Autodesk Inventor part; units mm, degrees
ref_plane "Work Plane1" through (0, 0, -15) normal (0, 0, 1) x (1, 0, 0)
ref_plane "YZ Plane" through (0, 0, 0) normal (1, 0, 0) x (0, 1, 0)
ref_plane "XZ Plane" through (0, 0, 0) normal (0, 1, 0) x (-1, 0, 0)
sketch "Sketch1" plane through (0, 0, 0) normal (0, 0, 1) x (1, 0, 0)
  line L0 (0, 0) -> (25, 0)
  line L1 (25, 0) -> (25, 40)
  line L2 (25, 40) -> (0, 40)
  line L3 (0, 40) -> (0, 0)
  dimension "d1" = 25
  dimension "d2" = 40
  dimension "d3" = 25
extrude "Extrusion1" add sketch "Sketch1" against normal blind 30
sketch "Sketch2" plane through (25, 0, 0) normal (1, 0, 0) x (0, 0, -1)
  line L0 (0, 0) -> (30, 0)
  circle A0 centre (15, 6.56) radius 2.46
extrude "Extrusion2" cut sketch "Sketch2" against normal blind 30
sketch "Sketch3" plane through (0, 0, 0) normal (-1, 0, 0) x (0, 0, 1)
  line L0 (0, 0) -> (-30, 0)
  line L1 (-25.05, 0) -> (-4.95, 0)
  line L2 (-4.95, 0) -> (-4.95, 33.12)
  line L3 (-4.95, 33.12) -> (-25.05, 33.12)
  line L4 (-25.05, 33.12) -> (-25.05, 0)
  dimension "d11" = 20.1
extrude "Extrusion3" cut sketch "Sketch3" against normal blind 20
sketch "Sketch4" plane through (0, 0, 0) normal (0, -1, 0) x (1, 0, 0)
  line L0 (20, -4.95) -> (20, -25.05)
  line L1 (20, -15) -> (25, -15)
  line L2 (25, 0) -> (25, -30)
  line L3 (20, -8.025) -> (25, -8.025)
  line L4 (25, -8.025) -> (25, -21.975)
  line L5 (25, -21.975) -> (20, -21.975)
  line L6 (20, -21.975) -> (20, -8.025)
  line L7 (20, -8.025) -> (25, -21.975) construction
  line L8 (25, -8.025) -> (20, -21.975) construction
  line L9 (25, -12.54) -> (25, -17.46)
  point P0 (0, 0)
  point P1 (22.5, -15)
  dimension "d14" = 13.95
extrude "Extrusion4" add sketch "Sketch4" along normal blind 15
sketch "Sketch5" plane through (20, 0, 0) normal (-1, 0, 0) x (0, 0, 1)
  circle A0 centre (-15, 6.56) radius 2.46
  circle A1 centre (-15, 6.56) radius 4.7025
  circle A2 centre (-15, 6.56) radius 2.46
  circle A3 centre (-15, 6.56) radius 2.46
  point P0 (0, 0)
  dimension "d17" = 9.405
extrude "Extrusion5" cut sketch "Sketch5" against normal blind 2.1
sketch "Sketch6" plane through (25, 0, 0) normal (1, 0, 0) x (0, 0, -1)
  circle A0 centre (15, 6.56) radius 4.7025
  line L0 (15, 6.56) -> (15, 23.56)
  circle A1 centre (15, 23.56) radius 2.46
  point P0 (0, 0)
  dimension "d20" = 17
  dimension "d21" = 4.92
extrude "Extrusion6" cut sketch "Sketch6" against normal blind 10 contours A1
sketch "Sketch7" plane through (20, 0, 0) normal (-1, 0, 0) x (0, 0, 1)
  circle A0 centre (-15, 23.56) radius 2.46
  circle A1 centre (-15, 23.56) radius 4.7025
  point P0 (0, 0)
  dimension "d24" = 9.405
extrude "Extrusion7" cut sketch "Sketch7" against normal blind 2.1
sketch "Sketch9" plane through (25, 0, 0) normal (1, 0, 0) x (0, 0, -1)
  circle A0 centre (15, 6.56) radius 2.46
  circle A1 centre (15, 6.56) radius 2.46
  circle A2 centre (15, 23.56) radius 2.46
  circle A3 centre (15, 23.56) radius 2.46
  line L0 (30, 40) -> (30, 0)
  line L1 (30, 0) -> (30, 40)
  line L2 (30, 40) -> (0, 40)
  line L3 (0, 40) -> (0, 0)
  line L4 (0, 0) -> (8.025, 0)
  line L5 (21.975, 0) -> (21.975, -15)
  line L6 (21.975, -15) -> (8.025, -15)
  line L7 (8.025, -15) -> (8.025, 0)
  line L8 (0, 0) -> (8.025, 0)
  line L9 (21.975, 0) -> (30, 0)
extrude "Extrusion8" add sketch "Sketch9" along normal blind 5
sketch "Sketch10" plane through (0, 40, 0) normal (0, 1, 0) x (1, 0, 0)
  line L0 (0, 30) -> (30, 30)
  line L1 (30, 0) -> (0, 0)
  line L2 (0, 30) -> (30, 30)
  line L3 (30, 30) -> (30, 0)
  line L4 (30, 0) -> (0, 0)
  line L5 (0, 0) -> (0, 30)
extrude "Extrusion9" add sketch "Sketch10" along normal blind 30
sketch "Sketch12" plane through (30, 0, 0) normal (1, 0, 0) x (0, 0, -1)
  circle A0 centre (15, 6.56) radius 2.46
  line L0 (15, 6.56) -> (15, 15.06)
  circle A1 centre (15, 15.06) radius 2.525
  point P0 (0, 0)
  dimension "d31" = 8.5
  dimension "d33" = 5.05
extrude "Extrusion10" cut sketch "Sketch12" against normal blind 30 contours A1
sketch "Sketch14" plane through (0, 0, 0) normal (0, 0, 1) x (1, 0, 0)
  line L0 (30, 70) -> (0, 70)
  line L1 (0, 70) -> (0, 85)
  line L2 (-15, 100) -> (-23, 100)
  line L3 (30, 0) -> (30, 70)
  line L4 (30, 118) -> (30, 70)
  arc A0 (0, 85) -> (-15, 100) centre (-15, 85) ccw
  line L5 (30, 105) -> (30, 100)
  line L6 (-23, 133) -> (15, 133)
  line L7 (-18, 130.5) -> (-23, 133)
  line L8 (-18, 130.5) -> (-13, 116.5)
  line L9 (-18, 102.5) -> (-23, 100)
  line L10 (-18, 102.5) -> (-13, 116.5)
  line L11 (30, 118) -> (15, 133)
  point P0 (0, 0)
  point P1 (0, 100)
  dimension "d47" = 30
  dimension "d54" = 15
extrude "Extrusion12" add sketch "Sketch14" against normal blind 30
sketch "Sketch15" plane through (0, 0, -25.05) normal (-1, 0, 0) x (0, 0, 1)
  line L0 (0, 33.12) -> (20.1, 33.12)
  line L1 (20.1, 33.12) -> (20.1, 0)
  line L2 (0, 33.12) -> (20.1, 33.12)
  line L3 (20.1, 33.12) -> (20.1, 31.1)
  line L4 (20.1, 31.1) -> (0, 31.1)
  line L5 (0, 31.1) -> (0, 33.12)
  point P0 (25.05, 0)
  dimension "d57" = 2.02
extrude "Extrusion13" add sketch "Sketch15" against normal blind 20
sketch "Sketch21" plane through (0, 0, 0) normal (0, 0, 1) x (1, 0, 0)
  arc A0 (0, 85) -> (-15, 100) centre (-15, 85) ccw
  arc A1 (0, 85) -> (-15, 100) centre (-15, 85) ccw
  line L0 (-15, 100) -> (-23, 100)
  line L1 (-15, 100) -> (-23, 100)
  line L2 (-23, 100) -> (-18, 102.5)
  line L3 (-23, 100) -> (-18, 102.5)
  line L4 (-18, 102.5) -> (-13, 116.5)
  line L5 (-18, 102.5) -> (-13, 116.5)
  line L6 (-13, 116.5) -> (-18, 130.5)
  line L7 (-13, 116.5) -> (-18, 130.5)
  line L8 (-18, 130.5) -> (-23, 133)
  line L9 (-18, 130.5) -> (-23, 133)
  line L10 (-23, 133) -> (15, 133)
  line L11 (-23, 133) -> (15, 133)
  line L12 (15, 133) -> (30, 118)
  line L13 (15, 133) -> (30, 118)
  line L14 (0, 85) -> (30, 85)
  line L15 (30, 85) -> (30, 118)
  point P0 (0, 0)
extrude "Extrusion14" add sketch "Sketch21" along normal blind 45
ref_plane "Work Plane1" through (0, 0, -15) normal (0, 0, 1) x (1, 0, 0)
mirror "Mirror1" about plane through (0, 0, -15) normal (0, 0, 1) of "Extrusion14"
properties part number "28mm_x_120mm"
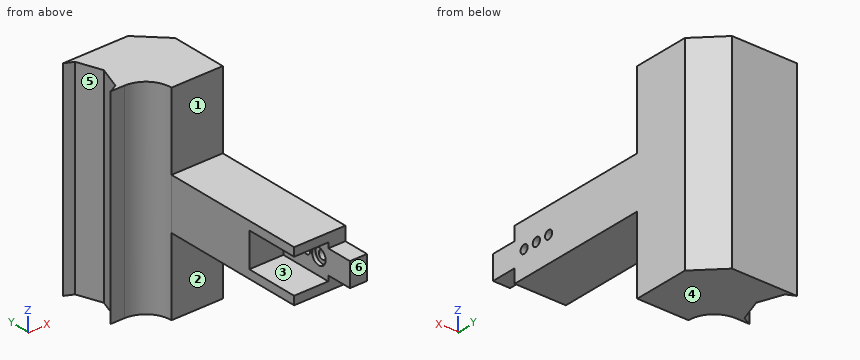
Work out the finished part from the listing and answer in its coordinate system (mm). Face numbers are marked on the shaded views. A direction names the side the tool comes from. Round coordinates to 2 decimals unless told otherwise and drop trailing zeros. Write each loop counter-clockwise with the first axis right and the second up, starting at its lowest first coordinate (ties: lowest second). Pieces come first, ordered by that corner, then holes. Notation, with made-up numbers: (32, 88) -> (75, 88) arc R28 ccw to (75, 124) -> close; hole circle Ø7 at (48, 30). An arc over 180 degrees is marked (long way). Write each question's results on one line, items separated by ' | '.
Q1. Section B-B, the plane y = 23.56 is taken. Write down the section's boundary in (x, z).
Data:
outline: (0, -30) -> (30, -30) -> (30, -17.46) -> (22.1, -17.46) -> (22.1, -19.7) -> (20, -19.7) -> (20, -25.05) -> (0, -25.05) -> close; (0, -4.95) -> (20, -4.95) -> (20, -10.3) -> (22.1, -10.3) -> (22.1, -12.54) -> (30, -12.54) -> (30, 0) -> (0, 0) -> close
Q2. Flat-ended cylindrical pins translate along their axes: P1, Ø8.5, axis at y = 23.56, z = -15, coming from the +X side; P2, Ø24, axis at x = 11, y = 21.5, coming from the +Z side; P3, Ø4.5, axis at y = 7, z = -13, coming from the -X side; P4, Ø3, axis at x = 9.5, y = 68, coming from the -Z side. Find the tip coordinate at first contact, or state that the pin passes through.
Data:
P1: x = 30 | P2: z = 0 | P3: x = 22.1 | P4: z = -30
Q3. Which of the six approach directions +Z, -Z, +X, -X, +Y, -Y give full straight-line access (tool end or side, diameter ignored) to the marked faces 1, 2 and 3?
Data:
face 1: +Z, +X, -X, -Y | face 2: -Z, +X, -X, -Y | face 3: -X, -Y
Q4. Determine the mould class of the marked faces 4, 5 and 6 for opening direction Y: released by +Y, released by -Y, zero draft, split by the parting line, or undercut.
Data:
face 4: zero draft | face 5: undercut | face 6: released by -Y
Q5. Section A-A, the plane z = -15 is taken. Give the number of separate pieces and of enclosed holes in the cut face, then the cut area to 3 significant figures.
Data:
separate pieces: 4 | enclosed holes: 0 | area: 3,820 mm^2
Q6. Straight lines are drawn through the part: line 1 along Y through (x, z) = (27, -15) (3 decimals); line 2 along Y through (x, z) = (20.4, -15) (1 decimal); line 3 along Z through (x, y) = (24.25, 15.06) (3 decimals). For each, find the intervals that lie inside material, in ascending order. Write a range as [from, to].
Data:
line 1: [-15, 4.1], [9.02, 12.535], [17.585, 21.1], [26.02, 121] | line 2: [-15, 1.9], [11.3, 12.5], [17.6, 18.9], [28.3, 127.6] | line 3: [-30, -17.525], [-12.475, 0]
Q7. Section C-C, the plane z = 26.5 is taken. Write down the section's boundary in (x, y).
Data:
outline: (-23, 100) -> (-15, 100) arc R15 cw to (0, 85) -> (30, 85) -> (30, 118) -> (15, 133) -> (-23, 133) -> (-18, 130.5) -> (-13, 116.5) -> (-18, 102.5) -> close
Q8. Section D-D, the plane y = 54 is taken. Write down the section's boundary in (x, z).
Data:
outline: (0, -30) -> (30, -30) -> (30, 0) -> (0, 0) -> close
